from build123d import *

# Parameters (mm, degrees)
SKETCH1_W               = 60
SKETCH1_H               = 60
BOSS_EXTRUDE1_DEPTH     = 260
CUT_EXTRUDE1_DEPTH      = 274.495886624
CUT_EXTRUDE1_DEPTH_BACK = 274.495886624
SKETCH2_R               = 7.5
CUT_EXTRUDE2_START      = 60
SKETCH3_R               = 15
CUT_EXTRUDE2_DEPTH      = 14
SKETCH4_W               = 20
SKETCH4_H               = 60
CUT_EXTRUDE3_DEPTH      = 5
CUT_EXTRUDE4_DEPTH      = 274.495886624
CUT_EXTRUDE4_DEPTH_BACK = 274.495886624
SKETCH5_R               = 2.6
CUT_EXTRUDE5_START      = -10
CUT_EXTRUDE5_DEPTH      = 4


with BuildPart() as part:
    # Sketch1 → Boss-Extrude1 (new body)
    with BuildSketch(Plane(origin=(0, 0, 0), x_dir=(0, 0, -1), z_dir=(1, 0, 0))):
        with Locations((30, 30)):
            Rectangle(SKETCH1_W, SKETCH1_H)
    extrude(amount=BOSS_EXTRUDE1_DEPTH)

    # Sketch2 → Cut-Extrude1 (cut, two sides: drawn at the far end of the back side and taken through both)
    with BuildSketch(Plane(origin=(0, 0, 0), x_dir=(1, 0, 0), z_dir=(0, 1, 0)).offset(-CUT_EXTRUDE1_DEPTH_BACK)):
        with Locations(Location((30, 30, 0), (0, 0, 270))):
            Circle(SKETCH2_R)
        with Locations(Location((230, 30, 0), (0, 0, 270))):
            Circle(SKETCH2_R)
    extrude(amount=CUT_EXTRUDE1_DEPTH + CUT_EXTRUDE1_DEPTH_BACK, mode=Mode.SUBTRACT)

    # Sketch3 → Cut-Extrude2 (cut)
    with BuildSketch(Plane(origin=(0, 0, 0), x_dir=(1, 0, 0), z_dir=(0, 1, 0)).offset(CUT_EXTRUDE2_START)):
        with Locations(Location((30, 30, 0), (0, 0, 90))):
            Circle(SKETCH3_R)
        with Locations(Location((230, 30, 0), (0, 0, 90))):
            Circle(SKETCH3_R)
    extrude(amount=-CUT_EXTRUDE2_DEPTH, mode=Mode.SUBTRACT)

    # Sketch4 → Cut-Extrude3 (cut)
    with BuildSketch(Plane.XY):
        with Locations((15, 30)):
            Rectangle(SKETCH4_W, SKETCH4_H)
        with Locations((245, 30)):
            Rectangle(SKETCH4_W, SKETCH4_H)
    cut_extrude3 = extrude(amount=-CUT_EXTRUDE3_DEPTH, mode=Mode.SUBTRACT)

    # Sketch5 → Cut-Extrude4 (cut, two sides: drawn at the far end of the back side and taken through both)
    with BuildSketch(Plane.XY.offset(-CUT_EXTRUDE4_DEPTH_BACK)):
        with Locations((15, 20)):
            Circle(SKETCH5_R)
        with Locations((15, 40)):
            Circle(SKETCH5_R)
        with Locations((245, 40)):
            Circle(SKETCH5_R)
        with Locations((245, 20)):
            Circle(SKETCH5_R)
    extrude(amount=CUT_EXTRUDE4_DEPTH + CUT_EXTRUDE4_DEPTH_BACK, mode=Mode.SUBTRACT)

    # Mirror2: Cut-Extrude3 across plane
    add(cut_extrude3.mirror(Plane.XY.offset(-30)), mode=Mode.SUBTRACT)

    # Sketch6 → Cut-Extrude5 (cut)
    with BuildSketch(Plane.XY.offset(CUT_EXTRUDE5_START)):
        Polygon((11, 20), (11, 0), (19, 0), (19, 20), (17, 23.464101615), (13, 23.464101615), align=None)
        Polygon((19, 60), (19, 40), (17, 36.535898385), (13, 36.535898385), (11, 40), (11, 60), align=None)
        Polygon((249, 40), (249, 60), (241, 60), (241, 40), (243, 36.535898385), (247, 36.535898385), align=None)
        Polygon((241, 0), (241, 20), (243, 23.464101615), (247, 23.464101615), (249, 20), (249, 0), align=None)
    cut_extrude5 = extrude(amount=-CUT_EXTRUDE5_DEPTH, mode=Mode.SUBTRACT)

    # Mirror3: Cut-Extrude5 across plane
    add(cut_extrude5.mirror(Plane.XY.offset(-30)), mode=Mode.SUBTRACT)


solid = part.part
Work out the finished part from the listing and answer in its coordinate system (mm). A direction names the side the tool comes from. Round coordinates to 2 decimals unless told otherwise and drop trailing zeros. Write each loop counter-clockwise with the first axis right and the second up, starting at its lowest first coordinate (ties: lowest second). Pieces come first, ordered by that corner, then holes. Notation, with made-up numbers: (48, -21) - (99, -21) arc R20 ccw to (99, -5) - close; hole circle Ø9 at (36.5, -14.75). An arc over 180 degrees is marked (long way). Answer in a Markdown table with one row per item. Add a question column.
1. For faces 1 (the flat face through (245, 9, -46)), 2 (the flat face through (255, 30, -2)), 3 (the flat face through (15, 48, -10)), determine the directions among +Z, -Z, +X, -X, +Y, -Y from which every point of the face is accessible in a straight line to the end or side of a thin tool.
2. Given pin 1 (4 mm diameter, centred on y = 34, z = -58.5, fed in from -X); pin 2 (6 mm diameter, centred on x = 15, y = 40, fed in from -Z); pin 3 (9 mm diameter, centred on x = 244, y = 9, fed in from +Z), each flat-ended and moving along its own axis, determine where each tip first touches the part or whether it passes through.
3. A cutting plane is placed at A-A, the plane x = 230. Determine the outline of the cut face in (y, z).
4. Find the intervals of material crossed by line 1 along Y through (x, z) = (15, -8.25); line 2 along X through (y, z) = (54.25, -30); line 3 along X through (y, z) = (40, -8), in increasing order. Write a range as from..to.
5. A cutting plane is placed at C-C, the plane y = 28.5. Determine the outline of the cut face in (x, z).
6. The mould has two halves that part along X. Classify faces 4 (the flat face through (129, 30, -60)), 5 (the flat face through (245, 9, -50)): +X half, -X half, draft (parallel to the pull), parting line (faces both ways), or undercut.
7. A cutting plane is placed at D-D, the plane y = 54.5. Count the separate pieces of the cut face and the enclosed holes in it, and give its area (3 significant figures).
8. A cutting plane is placed at B-B, the plane z = -30. Determine the outline of the cut face in (x, y).
Worked out:
| question | item | result |
|---|---|---|
| 1 | face 1 | -Y |
| 1 | face 2 | +Z, +Y, -Y |
| 1 | face 3 | +Y |
| 2 | pin 1 | x = 0 |
| 2 | pin 2 | z = -55 |
| 2 | pin 3 | z = -5 |
| 3 | outline | (0, -60) - (60, -60) - (60, -45) - (46, -45) - (46, -37.5) - (0, -37.5) - close; (0, -22.5) - (46, -22.5) - (46, -15) - (60, -15) - (60, 0) - (0, 0) - close |
| 4 | line 1 | 0..17.4, 22.6..37.4, 42.6..60 |
| 4 | line 2 | 0..15, 45..215, 245..260 |
| 4 | line 3 | 0..12.4, 17.6..242.4, 247.6..260 |
| 5 | outline | (0, -60) - (5, -60) - (5, -55) - (25, -55) - (25, -60) - (235, -60) - (235, -55) - (255, -55) - (255, -60) - (260, -60) - (260, 0) - (255, 0) - (255, -5) - (235, -5) - (235, 0) - (25, 0) - (25, -5) - (5, -5) - (5, 0) - (0, 0) - close; hole circle Ø15 at (30, -30); hole circle Ø15 at (230, -30) |
| 6 | face 4 | draft |
| 6 | face 5 | undercut |
| 7 | separate pieces | 1 |
| 7 | enclosed holes | 6 |
| 7 | area | 13,700 mm^2 |
| 8 | outline | (0, 0) - (22.5, 0) - (22.5, 46) - (15, 46) - (15, 60) - (0, 60) - close; (37.5, 0) - (222.5, 0) - (222.5, 46) - (215, 46) - (215, 60) - (45, 60) - (45, 46) - (37.5, 46) - close; (237.5, 0) - (260, 0) - (260, 60) - (245, 60) - (245, 46) - (237.5, 46) - close; hole circle Ø5.2 at (15, 20); hole circle Ø5.2 at (15, 40); hole circle Ø5.2 at (245, 20); hole circle Ø5.2 at (245, 40) |
